Answer from the drawing. Dimensions are ordinates in mm from the lowest x, y and z of the part. A direction names the side the tool comes from. Round coordinates to 2 decimals unless told otherwise and drop trailing zeros. Write each loop counter-clockwise with the first axis right and the second up, starting at its lowest first coordinate (ties: lowest second). Pieces come first, ordered by that corner, then holes. Notation, with made-up numbers: (30.5, 56) - (58.5, 56) arc R29 cw to (58.5, 91) - close; hole circle Ø3 at (78, 15.25). An arc over 180 degrees is marked (long way). Use a Markdown table: item, result. Add a question column.
1) A cutting plane is placed at A-A (x = 9). Give the vertices of the cut face in (y, z).
2) Find the intervals of material crossed by probe 1 along Z at (x, y) = (9, 38.6); probe 2 along Y at (x, z) = (17.25, 55); probe 3 along Y at (x, z) = (4.25, 47), in increasing order. Write a range as from..to.
3) Each of these flat-tipped pins is pushed along its axis until it touches: P1, Ø4, axis at x = 11, z = 55, coming from the +Y side; P2, Ø9, axis at x = 10.5, y = 22.5, coming from the +Z side; P3, Ø2, axis at x = 3.5, z = 13, coming from the -Y side. Where does it stop, or does it pass through?
4) A cutting plane is placed at C-C (y = 12.5). Give the vertices of the cut face in (x, z), then the cut area to 3 significant figures.
5) A cutting plane is placed at B-B (z = 57.25). Give the vertices of the cut face in (x, y).
6) A tool of negligible diameter and unlimited length cuts with its end or side. For the marked faces 4, 5 and 6, from which of +Z, -Z, +X, -X, +Y, -Y can it reach the whole face along a straight path? Write none if from no direction.
7) Determine the mould class of the marked faces 1, 2 and 3 for opening direction Y: +Y half, -Y half, draft (parallel to the pull), parting line (faces both ways), or undercut.
8) A cutting plane is placed at D-D (x = 16). Give the vertices of the cut face in (y, z), then the cut area to 3 significant figures.
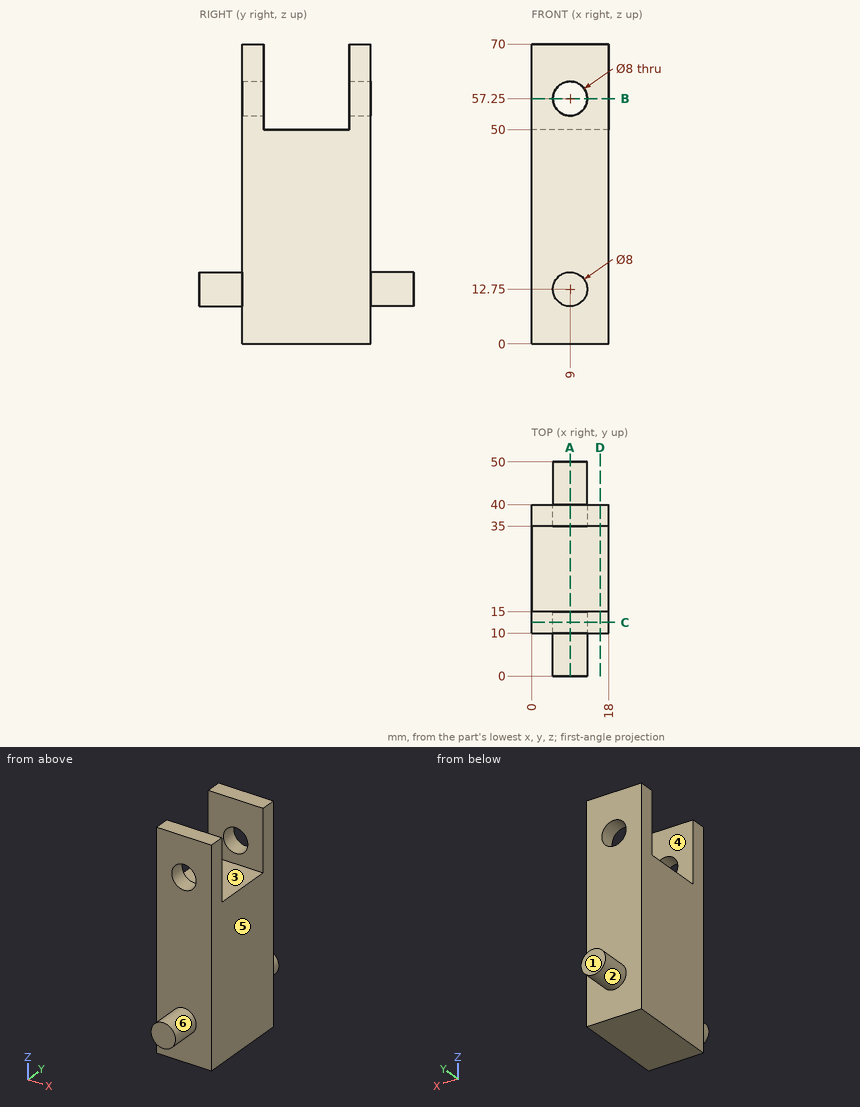
Entries:
| question | item | result |
|---|---|---|
| 1 | outline | (0, 8.75) - (10, 8.75) - (10, 0) - (40, 0) - (40, 8.75) - (50, 8.75) - (50, 16.75) - (40, 16.75) - (40, 53.25) - (35, 53.25) - (35, 50) - (15, 50) - (15, 53.25) - (10, 53.25) - (10, 16.75) - (0, 16.75) - close; (10, 61.25) - (15, 61.25) - (15, 70) - (10, 70) - close; (35, 61.25) - (40, 61.25) - (40, 70) - (35, 70) - close |
| 2 | probe 1 | z = 0..53.25, 61.25..70 |
| 2 | probe 2 | y = 10..15, 35..40 |
| 2 | probe 3 | y = 10..40 |
| 3 | P1 | stops at y = 40 |
| 3 | P2 | stops at z = 50 |
| 3 | P3 | stops at y = 10 |
| 4 | outline | (0, 0) - (18, 0) - (18, 70) - (0, 70) - close; hole circle Ø8 at (9, 57.25) |
| 4 | area | 1,210 mm² |
| 5 | outline | (0, 10) - (5, 10) - (5, 15) - (0, 15) - close; (0, 35) - (5, 35) - (5, 40) - (0, 40) - close; (13, 10) - (18, 10) - (18, 15) - (13, 15) - close; (13, 35) - (18, 35) - (18, 40) - (13, 40) - close |
| 6 | face 4 | +Z, +X, -X |
| 6 | face 5 | +Z, -Z, +X, +Y, -Y |
| 6 | face 6 | -Y |
| 7 | face 1 | +Y half |
| 7 | face 2 | draft |
| 7 | face 3 | undercut |
| 8 | outline | (10, 0) - (40, 0) - (40, 70) - (35, 70) - (35, 50) - (15, 50) - (15, 70) - (10, 70) - close |
| 8 | area | 1,700 mm² |
